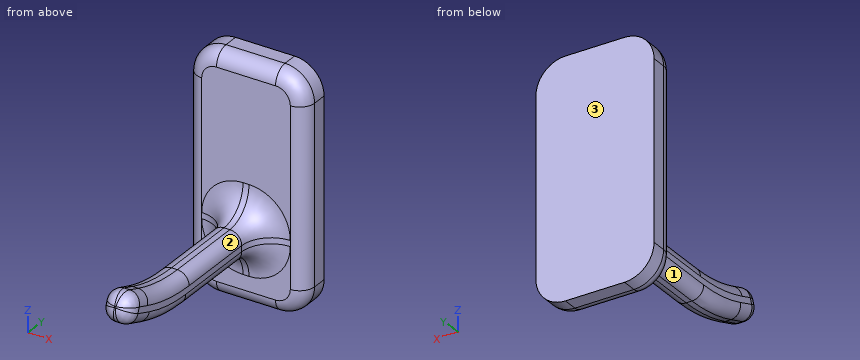
Autodesk Fusion 360 part; units mm, degrees
sketch "Sketch1" plane through (0, 0, 0) normal (1, 0, 0) x (0, 1, 0) in component "Main"
  line L0 (0, 0) -> (-5, 0)
  line L1 (-5, 0) -> (-5, 10)
  line L2 (-5, 10) -> (-30, 10)
  line L3 (-29.1184, 15) -> (-5, 15)
  line L4 (-5, 15) -> (-5, 40)
  line L5 (-5, 40) -> (0, 40)
  line L6 (0, 40) -> (0, 0)
  line L7 (-29.1184, 15) -> (-38.5153, 18.4202)
  line L8 (-30, 10) -> (-40.2254, 13.7217)
  line L9 (-38.5153, 18.4202) -> (-40.2254, 13.7217)
  line L10 (-5, 15) -> (-5, 10)
  dimension "d1" = 5
  dimension "d3" = 40
  dimension "d4" = 10
  dimension "d5" = 5
  dimension "d6" = 5
  dimension "d7" = 160
  dimension "d8" = 25
  dimension "d9" = 10
extrude "Extrude1" add sketch "Sketch1" along normal mid plane 5 contours L2 L3 L7 L8 L9 L10 in component "Main"
extrude "Extrude2" add sketch "Sketch1" along normal mid plane 20 contours L0 L1 L4 L5 L6 L10 in component "Main"
fillet "Fillet4" radius 30 2 edges at (0, -29.1184, 15) (0, -30, 10) in component "Main"
fillet "Fillet5" radius 2 12 edges at (-2.5, -14.4143, 15) (-2.5, -29.038, 15.4558) (-2.5, -36.3022, 17.6147) (2.5, -36.3022, 17.6147) (2.5, -29.038, 15.4558) (2.5, -14.4143, 15) (2.5, -14.8551, 10) (2.5, -29.9196, 10.4558) (2.5, -37.5981, 12.7655) (-2.5, -37.5981, 12.7655) (-2.5, -29.9196, 10.4558) (-2.5, -14.8551, 10) in component "Main"
fillet "Fillet6" radius 5 8 edges at (-1.9142, -5, 10.5858) (0, -5, 10) (1.9142, -5, 10.5858) (2.5, -5, 12.5) (1.9142, -5, 14.4142) (0, -5, 15) (-1.9142, -5, 14.4142) (-2.5, -5, 12.5) in component "Main"
fillet "Fillet7" radius 5 4 edges at (-10, -2.5, 40) (10, -2.5, 40) (10, -2.5, 0) (-10, -2.5, 0) in component "Main"
fillet "Fillet8" radius 2.5 8 edges at (-8.5355, -5, 38.5355) (-10, -5, 20) (-8.5355, -5, 1.4645) (0, -5, 0) (8.5355, -5, 1.4645) (10, -5, 20) (8.5355, -5, 38.5355) (0, -5, 40) in component "Main"
fillet "Fillet9" radius 2.4 8 edges at (2.5, -39.3703, 16.071) (1.9142, -40.025, 14.2722) (0, -40.2254, 13.7217) (-1.9142, -40.025, 14.2722) (-2.5, -39.3703, 16.071) (-1.9142, -38.7156, 17.8697) (0, -38.5153, 18.4202) (1.9142, -38.7156, 17.8697) in component "Main"
component "Main" placed x (1, 0, 0) y (0, 1, 0) z (0, 0, 1) at (0, 0, 0)
For this review, take the finished solid that the model builds, in its own axes (mm). Face numbers are marked on the shaded views. Round coordinates to 2 decimals unless told otherwise and drop trailing zeros. Write each loop counter-clockwise with the first axis right and the second up, starting at its lowest first coordinate (ties: lowest second). Pieces come first, ordered by that corner, then holes. Notation, with made-up numbers: (65.25, 62.25) -> (87.25, 62.25) arc R31 ccw to (87.25, 93.25) -> close; hole circle Ø8 at (40, -12). An arc over 180 degrees is marked (long way). One line per question, with ' | ' between items. Start each with the question number.
(1) Add section A-A, the plane y = -21. Write out the cut boundary in (x, z).
(2) Add section B-B, the plane z = 24. Write out the cut boundary in (x, y), plus the area to 3 significant figures.
(3) Mouldability with a two-part tool opening along Y and no side actions: class the marked faces 1, 2 and 3 as released by +Y, released by -Y, zero draft, split by the parting line, or undercut.
(4) For line 1 along Y through (x, z) = (-5, 24); line 2 along Y through (x, z) = (9.25, 26); line 3 along Z through (x, y) = (-0.75, -18.5), list the stretches that pass through material, from the lowest coordinate up. Write a range as from..to.
(5) Add section C-C, the plane y = -9. Write out the cut boundary in (x, z).
(6) Insertion check: P1, Ø3, axis at y = -14, z = 10, coming from the +X side; P2, Ø1.1, axis at x = 0, y = -15, coming from the +Z side; P3, Ø6, axis at y = -25, z = 8, coming from the +X side. Each pin has a flat end and moves straight along its axis. Give the tip position at first contact, or say it passes through.
Answer list:
1) outline: (-2.5, 12) arc R2 ccw to (-0.5, 10) -> (0.5, 10) arc R2 ccw to (2.5, 12) -> (2.5, 13) arc R2 ccw to (0.5, 15) -> (-0.5, 15) arc R2 ccw to (-2.5, 13) -> close
2) outline: (-10, -2.5) arc R2.5 ccw to (-7.5, -5) -> (7.5, -5) arc R2.5 ccw to (10, -2.5) -> (10, 0) -> (-10, 0) -> close | area: 97.3 mm²
3) face 1: zero draft | face 2: undercut | face 3: released by +Y
4) line 1: -5..0 | line 2: -4.29..0 | line 3: 10.02..14.98
5) outline: (-2.6, 12) arc R2.1 ccw to (-0.5, 9.9) -> (0.5, 9.9) arc R2.1 ccw to (2.6, 12) -> (2.6, 13) arc R2.1 ccw to (0.5, 15.1) -> (-0.5, 15.1) arc R2.1 ccw to (-2.6, 13) -> close
6) P1: x = 2.44 | P2: z = 15 | P3: x = 2.23
